Autodesk Inventor part; units mm, degrees
ref_plane "Work Plane2" through (-12.1066, 0, 34) normal (0, 0, 1) x (1, 0, 0)
ref_plane "YZ Plane" through (0, 0, 0) normal (1, 0, 0) x (0, 1, 0)
ref_plane "XZ Plane" through (0, 0, 0) normal (0, 1, 0) x (-1, 0, 0)
sketch "Sketch1" plane through (0, 0, 0) normal (0, 1, 0) x (-1, 0, 0)
  line L0 (0, 0) -> (0, 68)
  line L1 (0, 0) -> (10.6066, -10.6066)
  line L2 (0, 68) -> (10.6066, 78.6066)
  line L3 (5, 63) -> (5, 5)
  line L4 (10.6066, 78.6066) -> (10.6066, 63)
  line L5 (10.6066, -10.6066) -> (10.6066, 5)
  line L6 (10.6066, 63) -> (5, 63)
  line L7 (10.6066, 5) -> (5, 5)
  line L8 (10.6066, 5) -> (12.1066, 5)
  line L9 (12.1066, 5) -> (12.1066, -10.6066)
  line L10 (12.1066, -10.6066) -> (10.6066, -10.6066)
  line L11 (10.6066, -10.6066) -> (10.6066, 5)
  line L12 (10.6066, 63) -> (12.1066, 63)
  line L13 (12.1066, 63) -> (12.1066, 78.6066)
  line L14 (12.1066, 78.6066) -> (10.6066, 78.6066)
  line L15 (10.6066, 78.6066) -> (10.6066, 63)
  dimension "d0" = 68
  dimension "d1" = 15
  dimension "d2" = 135
  dimension "d4" = 15
  dimension "d5" = 135
  dimension "d6" = 5
  dimension "d7" = 5
  dimension "d8" = 5
  dimension "d35" = 1.5
extrude "Extrusion1" add sketch "Sketch1" along normal blind 200
sketch "Sketch2" plane through (0, 0, 68) normal (0.7071, 0, 0.7071) x (0.7071, 0, -0.7071)
  line L0 (-15, 0) -> (0, 0) construction
  line L1 (-7.5, 0) -> (-7.5, 200) construction
  circle A0 centre (-7.5, 185) radius 3.45
  circle A1 centre (-7.5, 15) radius 3.45
  line L2 (-15, 200) -> (0, 200)
  point P0 (48.0833, 0)
  dimension "d11" = 6.9
  dimension "d12" = 6.9
  dimension "d13" = 15
  dimension "d14" = 15
extrude "Extrusion2" cut sketch "Sketch2" against normal blind 6
sketch "Sketch3" plane through (0, 0, 68) normal (1, 0, 0) x (0, 0, -1)
  ellipse E0 centre (-5.3033, 185) end of major axis (-5.3033, 181.55) minor radius 2.4395 construction
  ellipse E1 centre (73.3033, 185) end of major axis (73.3033, 188.45) minor radius 2.4395 construction
  line L0 (-5.3033, 185) -> (73.3033, 185) construction
  ellipse E2 centre (-5.3033, 15) end of major axis (-5.3033, 11.55) minor radius 2.4395 construction
  ellipse E3 centre (73.3033, 15) end of major axis (73.3033, 18.45) minor radius 2.4395 construction
  line L1 (-5.3033, 15) -> (73.3033, 15) construction
  line L2 (0, 200) -> (68, 200) construction
  line L3 (34, 200) -> (34, 0) construction
  line L4 (63, 0) -> (5, 0) construction
  line L5 (44, 200) -> (44, 0) construction
  line L6 (24, 200) -> (24, 0) construction
  circle A0 centre (44, 185) radius 2.6
  circle A1 centre (24, 185) radius 2.6
  circle A2 centre (24, 15) radius 2.6
  circle A3 centre (44, 15) radius 2.6
  point P0 (68, 0)
  dimension "d17" = 10
  dimension "d18" = 10
  dimension "d19" = 5.2
  dimension "d20" = 5.2
  dimension "d21" = 5.2
  dimension "d22" = 5.2
extrude "Extrusion3" cut sketch "Sketch3" against normal up to next
sketch "Sketch4" plane through (0, 0, 68) normal (1, 0, 0) x (0, 0, -1)
  line L0 (5, 0) -> (5, 200)
  line L1 (63, 0) -> (63, 200)
  line L2 (5, 170) -> (63, 170)
  line L3 (5, 30) -> (63, 30)
  circle A0 centre (24, 185) radius 2.6
  circle A1 centre (24, 15) radius 2.6
  point P0 (68, 0)
  dimension "d25" = 15
  dimension "d26" = 15
extrude "Extrusion4" cut sketch "Sketch4" against normal up to next contours L0 L2 L1 L3
sketch "Sketch5" plane through (0, 0, 68) normal (1, 0, 0) x (0, 0, -1)
  circle A0 centre (24, 185) radius 2.6
  circle A1 centre (24, 185) radius 4.75
  circle A2 centre (44, 185) radius 2.6
  circle A3 centre (44, 185) radius 4.75
  circle A4 centre (24, 15) radius 2.6
  circle A5 centre (24, 15) radius 4.75
  circle A6 centre (44, 15) radius 2.6
  circle A7 centre (44, 15) radius 4.75
  point P0 (68, 0)
  dimension "d29" = 9.5
  dimension "d30" = 9.5
  dimension "d31" = 9.5
  dimension "d32" = 9.5
extrude "Extrusion5" cut sketch "Sketch5" against normal blind 3
ref_plane "Work Plane2" through (-12.1066, 0, 34) normal (0, 0, 1) x (1, 0, 0)
mirror "Mirror2" about plane through (-12.1066, 0, 34) normal (0, 0, 1) of "Extrusion2"
equation "\"d4\" = d1"
equation "\"d5\" = d2"
equation "\"d12\" = d11"
equation "\"d14\" = d13"
equation "\"d20\" = d19"
equation "\"d21\" = d19"
equation "\"d22\" = d19"
equation "\"d30\" = d29"
equation "\"d31\" = d29"
equation "\"d32\" = d29"
properties part number "Z Axis Cover Frame"
Verification items for the finished model (mm, model axes). A direction names the side the tool comes from. Coordinates: 2 decimals unless noted, no trailing zeros. Write each loop counter-clockwise with the first axis right and the second up, starting at its lowest first coordinate (ties: lowest second). Pieces come first, ordered by that corner, then holes. Notation, with made-up numbers: (-27.5, 41.5) - (14.5, 41.5) arc R20 ccw to (14.5, 46.5) - close; hole circle Ø4 at (33, 47.25). An arc over 180 degrees is marked (long way). Write item = value, one per line.
Q1. Access from +Z, -Z, +X, -X, +Y, -Y to the whole of each face (thin tool, end or side, straight path). Record for faces 3 (the face through (-2, 30, 34)), 4 (the face through (-9.513, 15.048, -1.025)), 5 (the face through (-1.48, 18.21, 47.5)), 6 (the face through (-6, 99, 5)).
Answer:
face_3 = +X, -X
face_4 = none
face_5 = +X
face_6 = -X
Q2. Cross-section at C-C (y = 95). Enter the section's corners in (x, z), plus the area to 3 significant figures.
Answer:
outline = (-12.11, -10.61) - (-10.61, -10.61) - (0, 0) - (0, 5) - (-12.11, 5) - close; (-12.11, 63) - (0, 63) - (0, 68) - (-10.61, 78.61) - (-12.11, 78.61) - close
area = 265 mm²
Q3. Cross-section at B-B (z = 14). Enter the section's corners in (x, y), plus the area to 3 significant figures.
Answer:
outline = (-5, 0) - (0, 0) - (0, 30) - (-5, 30) - close; (-5, 170) - (0, 170) - (0, 200) - (-5, 200) - close
area = 300 mm²
Q4. Cross-section at D-D (y = 15). Give the number of separate pieces and of enclosed holes in the cut face, plus the area to 3 significant figures.
Answer:
separate_pieces = 3
enclosed_holes = 0
area = 395 mm²
Q5. Mould release check, pull along Y, two halves, no side actions. Record for faces 1 (the face through (-9.58, 15.05, 69.09)), 2 (the face through (-5, 185, 34)): released by +Y, released by -Y, zero draft, split by the parting line, or undercut.
Answer:
face_1 = undercut
face_2 = zero draft
Q6. Material ranges on L1, parallel to Y at x = -3.75, z = 44; L2, parallel to Y at x = -1, z = 24; L3, parallel to Y at x = -1, z = 19, recorded low to high. Write a range as from..to.
Answer:
L1 = 0..12.4, 17.6..30, 170..182.4, 187.6..200
L2 = 0..10.25, 19.75..30, 170..180.25, 189.75..200
L3 = 0..30, 170..200
Q7. Go/stop test with flat-tipped pins: pin 1 Ø4 at (y, z) = (15, 44) entering from -X; pin 2 Ø5.5 at (y, z) = (15, 24) entering from +X; pin 3 Ø2 at (x, y) = (-4.5, 105) entering from -Z; pin 4 Ø2 at (x, y) = (-8.5, 46.5) entering from +Z. Record where each tip stops, or that it passes through.
Answer:
pin_1 = through
pin_2 = -3
pin_3 = -5.5
pin_4 = 77.5
Q8. Cross-section at A-A (z = 44). Enter the section's corners in (x, y).
Answer:
outline = (-5, 0) - (0, 0) - (0, 10.25) - (-3, 10.25) - (-3, 12.4) - (-5, 12.4) - close; (-5, 17.6) - (-3, 17.6) - (-3, 19.75) - (0, 19.75) - (0, 30) - (-5, 30) - close; (-5, 170) - (0, 170) - (0, 180.25) - (-3, 180.25) - (-3, 182.4) - (-5, 182.4) - close; (-5, 187.6) - (-3, 187.6) - (-3, 189.75) - (0, 189.75) - (0, 200) - (-5, 200) - close
